```python
from build123d import *

# Parameters (mm, degrees)
SKETCH1_R           = 50
BOSS_EXTRUDE1_DEPTH = 250
SKETCH2_W           = 25
SKETCH2_H           = 25
CUT_EXTRUDE1_DEPTH  = 175
FILLET1_R           = 12.5
FILLET2_R           = 12.5


with BuildPart() as part:
    # Sketch1 → Boss-Extrude1 (new body)
    with BuildSketch(Plane.XY):
        Circle(SKETCH1_R)
    extrude(amount=BOSS_EXTRUDE1_DEPTH)

    # Sketch2 → Cut-Extrude1 (cut)
    with BuildSketch(Plane.XY.offset(250)):
        with Locations((-0.919686695, 49.991541048)):
            Rectangle(SKETCH2_W, SKETCH2_H)
    extrude(amount=-CUT_EXTRUDE1_DEPTH, mode=Mode.SUBTRACT)

    # Fillet1
    fillet1_edges = [part.edges().sort_by_distance(p)[0] for p in [
        (-13.419686695, 42.828502974, 75),
    ]]
    fillet(fillet1_edges, radius=FILLET1_R)

    # Fillet2
    fillet2_edges = [part.edges().sort_by_distance(p)[0] for p in [
        (11.580313305, 43.066010777, 75),
    ]]
    fillet(fillet2_edges, radius=FILLET2_R - 0.0001)  # a hair under: the kernel refuses the full size


solid = part.part
```
For this review, take the finished solid that the model builds, in its own axes (mm). A direction names the side the tool comes from. Coordinates: 2 decimals unless noted, no trailing zeros. Write each loop counter-clockwise with the first axis right and the second up, starting at its lowest first coordinate (ties: lowest second). Pieces come first, ordered by that corner, then holes.
(1) For pin 1 Ø12.5 at (x, z) = (-7, 204.5) entering from +Y; pin 2 Ø2 at (y, z) = (-19.5, 64) entering from +X; pin 3 Ø8 at (x, z) = (-30.5, 154) entering from -Y, all flat-tipped, find the tip position at first contact; note any pin that passes through.
(2) The part is to be moulded in two halves that separate along Z. For faces 1 (the face through (11.58, 43, 170)), 2 (the face through (-1, 1, 0)), 3 (the face through (-1, 0, 250)), say which applies: +Z half, -Z half, draft (parallel to the pull), parting line (faces both ways), or undercut.
(3) Add section B-B on y = 35. Give the boundary of the cut face in (x, z), then the cut area to 3 significant figures.
(4) Add section A-A on z = 163.5. Give the boundary of the cut face in (x, y), then the cut area to 3 significant figures.
(5) Wall thickness on probe 1 along Y at (x, z) = (-1.5, 212); probe 2 along Y at (x, z) = (-13.5, 91); probe 3 along X at (y, z) = (-33.5, 22.5): over which ranges is each line inside the solid? List them lowest first.
(6) Tool access review of faces 4 (the face through (-9.855, 43.829, 78.759)), 5 (the face through (23.07, -44.36, 123.25)): name each direction out of +Z, -Z, +X, -X, +Y, -Y from which nothing blocks a thin tool from reaching the whole face with its end or side.
Answer sheet:
1. pin 1: stops at y = 37.49
1. pin 2: stops at x = 46.45
1. pin 3: stops at y = -42.4
2. face 1: draft
2. face 2: -Z half
2. face 3: +Z half
3. outline: (-35.71, 0) - (35.71, 0) - (35.71, 250) - (-35.71, 250) - close
3. area: 17,900 mm2
4. outline: (-13.42, 37.49) - (-13.42, 48.17) arc R50 ccw (long way) to (11.58, 48.64) - (11.58, 37.49) - close
4. area: 7,550 mm2
5. probe 1: y = -49.98 to 37.49
5. probe 2: y = -48.14 to 48.14
5. probe 3: x = -37.12 to 37.12
6. face 4: +Z, +Y
6. face 5: +Z, -Z
